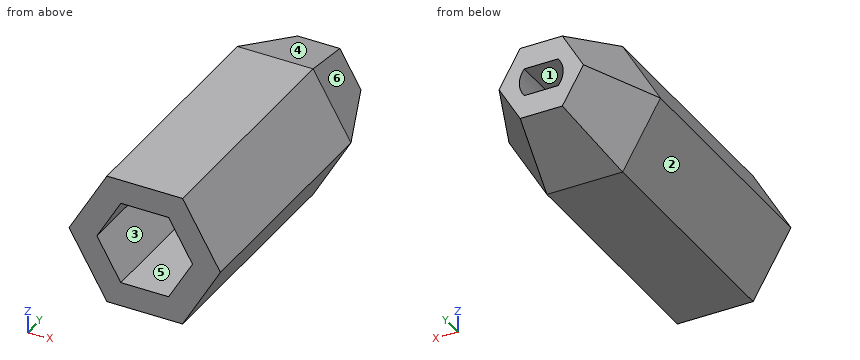
Autodesk Inventor part; units mm, degrees
ref_plane "YZ Plane" through (0, 0, 0) normal (1, 0, 0) x (0, 1, 0)
ref_plane "XZ Plane" through (0, 0, 0) normal (0, 1, 0) x (-1, 0, 0)
ref_plane "XY Plane" through (0, 0, 0) normal (0, 0, 1) x (1, 0, 0)
sketch "Boceto16" plane through (0, 0, 0) normal (0, 1, 0) x (-1, 0, 0)
  line L0 (0, 0) -> (6, 0)
  line L1 (6, 0) -> (3, -5.1962)
  line L2 (3, -5.1962) -> (-3, -5.1962)
  line L3 (-3, -5.1962) -> (-6, 0)
  line L4 (-6, 0) -> (-3, 5.1962)
  line L5 (-3, 5.1962) -> (3, 5.1962)
  line L6 (3, 5.1962) -> (6, 0)
  line L7 (6, 0) -> (9.5, 0)
  line L8 (9.5, 0) -> (4.75, -8.2272)
  line L9 (4.75, -8.2272) -> (-4.75, -8.2272)
  line L10 (-4.75, -8.2272) -> (-9.5, 0)
  line L11 (-9.5, 0) -> (-4.75, 8.2272)
  line L12 (-4.75, 8.2272) -> (4.75, 8.2272)
  line L13 (4.75, 8.2272) -> (9.5, 0)
  dimension "d55" = 6
  dimension "d56" = 3.5
extrude "Extrusión10" add sketch "Boceto16" along normal blind 30
sketch "Boceto17" plane through (0, 30, 0) normal (0, 1, 0) x (1, 0, 0)
  line L0 (-9.5, 0) -> (-4.75, -8.2272)
  line L1 (-9.5, 0) -> (-4.75, 8.2272)
  line L2 (-4.75, 8.2272) -> (4.75, 8.2272)
  line L3 (4.75, 8.2272) -> (9.5, 0)
  line L4 (9.5, 0) -> (4.75, -8.2272)
  line L5 (4.75, -8.2272) -> (-4.75, -8.2272)
  line L6 (-4.75, -8.2272) -> (-9.5, 0)
  point P0 (0, 0)
  point P1 (0, 0)
extrude "Extrusión11" add sketch "Boceto17" along normal blind 10 draft -20
sketch "Boceto18" plane through (0, 40, 0) normal (0, 1, 0) x (1, 0, 0)
  line L0 (0, 1.75) -> (2.1213, 1.75)
  line L1 (0, -1.75) -> (2.1213, -1.75)
  line L2 (0, -1.75) -> (-2.1213, -1.75)
  line L3 (0, 1.75) -> (-2.1213, 1.75)
  arc A0 (-2.1213, 1.75) -> (-2.1213, -1.75) centre (0, 0) ccw
  arc A1 (2.1213, -1.75) -> (2.1213, 1.75) centre (0, 0) ccw
extrude "Extrusión12" cut sketch "Boceto18" against normal blind 5
For this review, take the finished solid that the model builds, in its own axes (mm). Face numbers are marked on the shaded views. A direction names the side the tool comes from. Round coordinates to 2 decimals unless told otherwise and drop trailing zeros. Loops run counter-clockwise (first coordinate to the right, second up) from the corner with the lowest first, then second, coordinate; pieces in that order, holes last.
Q1. Add section C-C on z = -2.5. Write out the cut boundary in (x, y), plus the area to 3 significant figures.
Result sheet:
outline: (-8.06, 0) - (-4.56, 0) - (-4.56, 30) - (4.56, 30) - (4.56, 0) - (8.06, 0) - (8.06, 30) - (3.85, 40) - (-3.85, 40) - (-8.06, 30) - close
area: 329 mm2
Q2. Add section D-D on y = 32.5. Write out the cut boundary in (x, z).
Result sheet:
outline: (-8.45, 0) - (-4.22, -7.32) - (4.22, -7.32) - (8.45, 0) - (4.22, 7.32) - (-4.22, 7.32) - close
Q3. To check wall thickness, follow line 1 along Z through (x, y) = (0.75, 2); line 2 along X through (y, z) = (5, 0); line 3 along Y through (x, z) = (-1, -3.75). State the ranges of each line that lie inside material, in increasing order.
Result sheet:
line 1: z = -8.23 to -5.2, 5.2 to 8.23
line 2: x = -9.5 to -6, 6 to 9.5
line 3: y = 30 to 40
Q4. Mouldability with a two-part tool opening along X and no side actions: class the marked faces 4, 5 and 6 as +X half, -X half, draft (parallel to the pull), parting line (faces both ways), or undercut.
Result sheet:
face 4: draft
face 5: undercut
face 6: +X half
Q5. Add section B-B on x = -0.5. Write out the cut boundary in (y, z), plus the area to 3 significant figures.
Result sheet:
outline: (0, -8.23) - (30, -8.23) - (40, -4.59) - (40, -1.75) - (35, -1.75) - (35, 1.75) - (40, 1.75) - (40, 4.59) - (30, 8.23) - (0, 8.23) - (0, 5.2) - (30, 5.2) - (30, -5.2) - (0, -5.2) - close
area: 293 mm2
Q6. Insertion check: pin 1 Ø2 at (x, y) = (0.5, 38) entering from -Z; pin 2 Ø6 at (y, z) = (27, 6.5) entering from -X; pin 3 Ø1.3 at (x, y) = (-0.5, 36.5) entering from +Z. Each pin has a flat end and moves straight along its axis. Give the tip position at first contact, or say it passes through.
Result sheet:
pin 1: stops at z = -5.68
pin 2: stops at x = -7.48
pin 3: stops at z = 6.1
Q7. Machinability: for the marked faces 1, 2 and 3, which of the approach directions +Z, -Z, +X, -X, +Y, -Y give a long, thin tool a straight path to every point of the face, cutting with its end or side? Answer none if there is none.
Result sheet:
face 1: +Y
face 2: -Z, -X, +Y, -Y
face 3: -Y
Q8. Add section A-A on y = 20. Write out the cut boundary in (x, z), plus the area to 3 significant figures.
Result sheet:
outline: (-9.5, 0) - (-4.75, -8.23) - (4.75, -8.23) - (9.5, 0) - (4.75, 8.23) - (-4.75, 8.23) - close; hole (-6, 0) - (-3, -5.2) - (3, -5.2) - (6, 0) - (3, 5.2) - (-3, 5.2) - close
area: 141 mm2
